The figure shows three views and two pictorial views of one solid part (mm, origin at its lowest corner). Answer the questions. A direction names the side the tool comes from. Coordinates: 2 decimals unless noted, no trailing zeros. Write each loop counter-clockwise with the first axis right and the second up, starting at its lowest first coordinate (ties: lowest second). Pieces come first, ordered by that corner, then holes.
Item 1: A tool of negligible diameter and unlimited length cuts with its end or side. For the marked faces 1 and 2, from which of +Z, -Z, +X, -X, +Y, -Y can it reach the whole face along a straight path? Write none if from no direction.
Item 2: Straight lines are drawn through the part: probe 1 along Y at (x, z) = (101, 34); probe 2 along Y at (x, z) = (16, 152); probe 3 along X at (y, z) = (50.8, 17.5). For each, find the intervals that lie inside material, in ascending order.
Item 3: This flat-tipped pin is pushed along its axis until it touches: P1, Ø12, axis at x = 89, y = 47, coming from the +Z side. Where does it stop, or does it pass through?
Item 4: Section D-D (z = 104) is taken. Give the vertices of the cut face in (x, y).
Item 5: Section A-A (x = 101.6) is taken. Give the vertices of the cut face in (y, z), then the cut area to 3 significant figures.
Item 6: Section C-C (x = 68) is taken. Give the vertices of the cut face in (y, z), then the cut area to 3 significant figures.
Item 7: Section B-B (y = 25.5) is taken. Give the vertices of the cut face in (x, z).
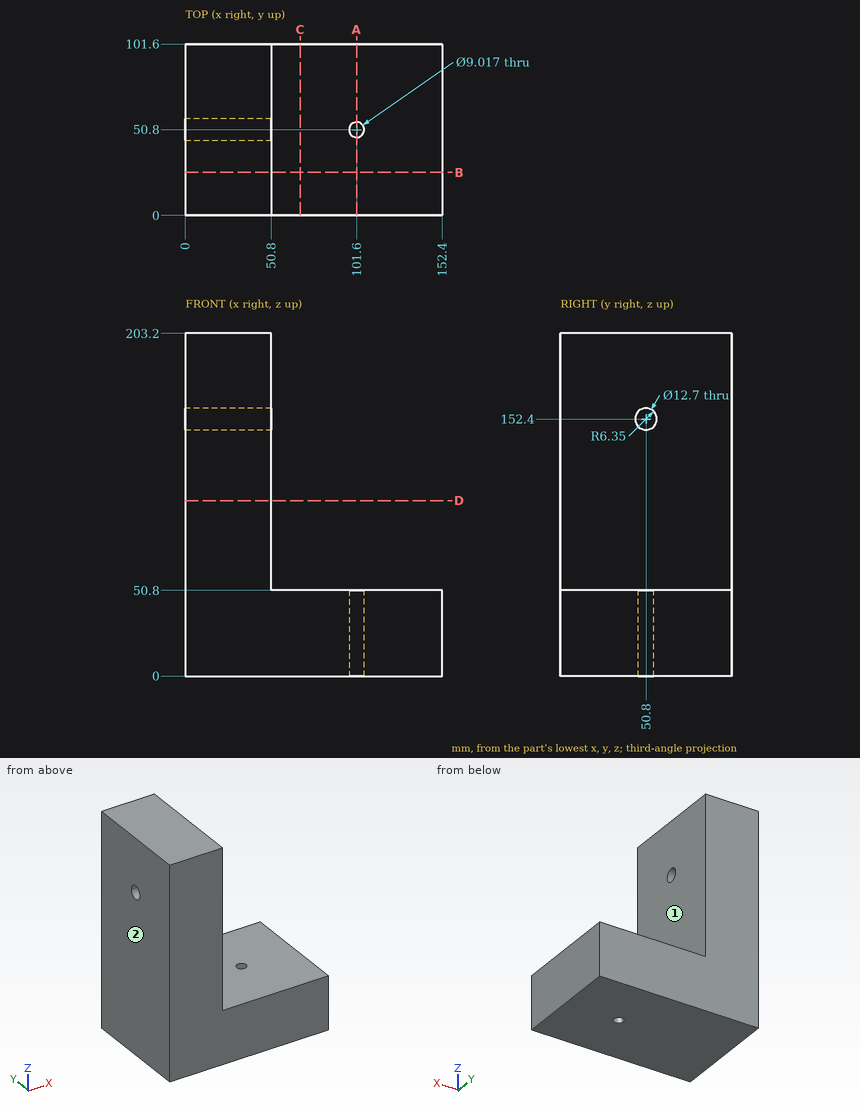
Established:
1. face 1: +Z, +X, +Y, -Y
1. face 2: +Z, -Z, -X, +Y, -Y
2. probe 1: y = 0 to 46.33, 55.27 to 101.6
2. probe 2: y = 0 to 44.46, 57.14 to 101.6
2. probe 3: x = 0 to 97.09, 106.11 to 152.4
3. P1: stops at z = 50.8
4. outline: (0, 0) - (50.8, 0) - (50.8, 101.6) - (0, 101.6) - close
5. outline: (0, 0) - (46.29, 0) - (46.29, 50.8) - (0, 50.8) - close; (55.31, 0) - (101.6, 0) - (101.6, 50.8) - (55.31, 50.8) - close
5. area: 4,700 mm2
6. outline: (0, 0) - (101.6, 0) - (101.6, 50.8) - (0, 50.8) - close
6. area: 5,160 mm2
7. outline: (0, 0) - (152.4, 0) - (152.4, 50.8) - (50.8, 50.8) - (50.8, 203.2) - (0, 203.2) - close
